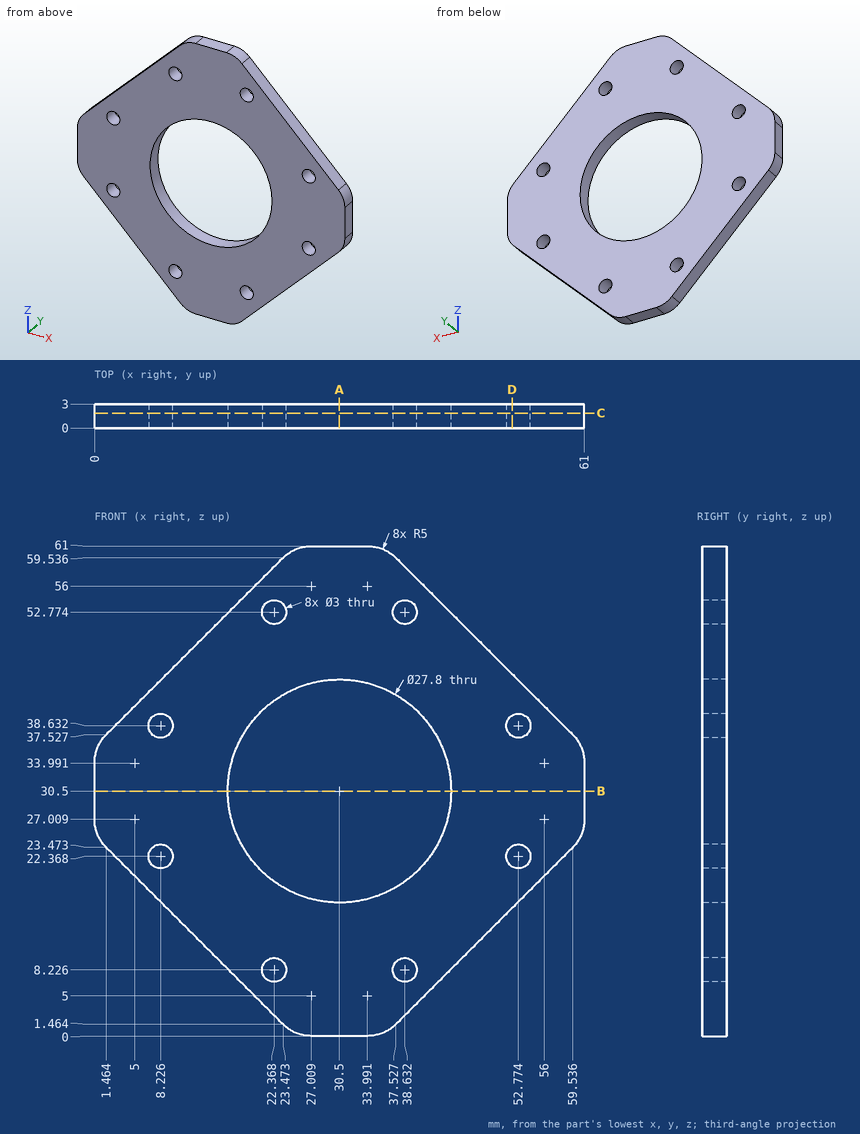
For this review, use the dimensioned drawing (mm, ordinates from the lowest corner) and the shaded views. Coordinates: 2 decimals unless noted, no trailing zeros. Order: outer loops, then holes, each group sorted by start corner. A loop starts at its lowest first (then second) coordinate and runs counter-clockwise, first axis right, second up. Notation, with made-up numbers: (3, 74) - (59, 74) arc R32 cw to (59, 109) - close; hole circle Ø11 at (44, 49.5). An arc over 180 degrees is marked (long way). Use one line per item in the form item = value.
Q1. Consider section A-A (x = 30.5). Give the boundary of the cut face in (y, z).
Checked values:
outline = (0, 0) - (3, 0) - (3, 16.6) - (0, 16.6) - close; (0, 44.4) - (3, 44.4) - (3, 61) - (0, 61) - close
Q2. For probe 1 along X at (y, z) = (2, 30.5); probe 2 along X at (y, z) = (2.2, 39) (1 decimal); probe 3 along X at (y, z) = (1.95, 9) (1 decimal), list the stretches that pass through material, from the lowest coordinate up. Write a range as from..to.
Checked values:
probe_1 = 0..16.6, 44.4..61
probe_2 = 2.9..6.8, 9.7..19.5, 41.5..51.3, 54.2..58.1
probe_3 = 15.9..21.1, 23.7..37.3, 39.9..45.1
Q3. Consider section B-B (z = 30.5). Give the boundary of the cut face in (x, y).
Checked values:
outline = (0, 0) - (16.6, 0) - (16.6, 3) - (0, 3) - close; (44.4, 0) - (61, 0) - (61, 3) - (44.4, 3) - close
Q4. Consider section C-C (y = 1.85). Give the number of separate pieces and of enclosed holes in the cut face, then the cut area to 3 significant figures.
Checked values:
separate_pieces = 1
enclosed_holes = 9
area = 1,810 mm2
Q5. For P1, Ø1, axis at y = 1, z = 15, coming from the -X side; P2, Ø10, axis at x = 12.5, z = 22, coming from the -Y side; P3, Ø2.5, axis at x = 52.77, z = 38.63, coming from the -Y side, all flat-tipped, find the tip position at first contact; note any pin that passes through.
Checked values:
P1 = 9.44
P2 = 0
P3 = through
Q6. Consider section D-D (x = 52). Give the boundary of the cut face in (y, z).
Checked values:
outline = (0, 15.94) - (3, 15.94) - (3, 21.08) - (0, 21.08) - close; (0, 23.65) - (3, 23.65) - (3, 37.35) - (0, 37.35) - close; (0, 39.92) - (3, 39.92) - (3, 45.06) - (0, 45.06) - close
